from build123d import *

# Parameters (mm, degrees)
SKETCH1_R               = 10
SKETCH1_R_2             = 6
BOSS_EXTRUDE1_DEPTH     = 3
SKETCH2_R               = 1.5
CUT_EXTRUDE1_DEPTH      = 4
CUT_EXTRUDE1_DEPTH_BACK = 4
F_4_0MM_DOWEL_HOLE1_D   = 4


with BuildPart() as part:
    # Sketch1 → Boss-Extrude1 (new body, symmetric)
    with BuildSketch(Plane(origin=(0, 0, 0), x_dir=(0, 0, -1), z_dir=(1, 0, 0))):
        Circle(SKETCH1_R)
        with BuildLine():
            ThreePointArc((40.6, -5.969924623), (34, 0), (40.6, 5.969924623))
            Line((40.6, 5.969924623), (1, 9.949874371))
            ThreePointArc((1, 9.949874371), (7.416198487, 6.708203932), (10, 0))
            ThreePointArc((10, 0), (7.416198487, -6.708203933), (1, -9.949874371))
            Line((1, -9.949874371), (40.6, -5.969924623))
        make_face()
        with Locations((40, 0)):
            Circle(SKETCH1_R_2)
    extrude(amount=BOSS_EXTRUDE1_DEPTH, both=True)

    # Sketch2 → Cut-Extrude1 (cut, two sides)
    with BuildSketch(Plane(origin=(0, 0, 0), x_dir=(0, 0, -1), z_dir=(1, 0, 0))) as cut_extrude1_sk:
        with Locations((4.949747468, 4.949747468)):
            Circle(SKETCH2_R)
        with Locations((4.949747468, -4.949747468)):
            Circle(SKETCH2_R)
        with Locations((-4.949747468, -4.949747468)):
            Circle(SKETCH2_R)
        with Locations((-4.949747468, 4.949747468)):
            Circle(SKETCH2_R)
    extrude(amount=CUT_EXTRUDE1_DEPTH, mode=Mode.SUBTRACT)
    extrude(cut_extrude1_sk.sketch, amount=-CUT_EXTRUDE1_DEPTH_BACK, mode=Mode.SUBTRACT)

    # 4.0mm Dowel Hole1 (through all)
    with Locations(Plane(origin=(3, 0, 0), x_dir=(0, 0, -1), z_dir=(1, 0, 0))):
        with Locations((40, 0)):
            Hole(F_4_0MM_DOWEL_HOLE1_D / 2)


solid = part.part
Input: part model. Units: mm. Frame: model coordinates. Round coordinates to 2 decimals unless told otherwise and drop trailing zeros. Order: outer loops, then holes, each group sorted by start corner. A loop starts at its lowest first (then second) coordinate and runs counter-clockwise, first axis right, second up.
1. Cut plane A-A, the plane y = 0. Output: boundary loops of the cut face in (x, z), then the cut area to 3 significant figures.
The answers:
outline: (-3, -46) - (3, -46) - (3, -42) - (-3, -42) - close; (-3, -38) - (3, -38) - (3, 10) - (-3, 10) - close
area: 312 mm2
2. Cut plane D-D, the plane x = 2.5. Output: boundary loops of the cut face in (y, z), then the cut area to 3 significant figures.
The answers:
outline: (-9.95, -1) - (-5.97, -40.6) arc R6 ccw to (5.97, -40.6) - (9.95, -1) arc R10 ccw (long way) to start; hole circle Ø3 at (-4.95, -4.95); hole circle Ø3 at (-4.95, 4.95); hole circle Ø4 at (0, -40); hole circle Ø3 at (4.95, -4.95); hole circle Ø3 at (4.95, 4.95)
area: 816 mm2
3. Cut plane B-B, the plane y = -4. Output: boundary loops of the cut face in (x, z), then the cut area to 3 significant figures.
The answers:
outline: (-3, -44.47) - (3, -44.47) - (3, -6.11) - (-3, -6.11) - close; (-3, -3.79) - (3, -3.79) - (3, 3.79) - (-3, 3.79) - close; (-3, 6.11) - (3, 6.11) - (3, 9.17) - (-3, 9.17) - close
area: 294 mm2
4. Material intervals for line 1 (Z direction, x = -2, y = 4.75); line 2 (Z direction, x = -1.75, y = 4); line 3 (Y direction, x = 2.75, z = -41.5), sorted ascending.
The answers:
line 1: z = -43.67 to -6.44, -3.46 to 3.46, 6.44 to 8.8
line 2: z = -44.47 to -6.11, -3.79 to 3.79, 6.11 to 9.17
line 3: y = -5.81 to -1.32, 1.32 to 5.81
5. Pin query (flat end, axial travel): P1, Ø3, axis at x = 2, z = -7, coming from the +Y side; P2, Ø3, axis at x = 1.5, y = 4, coming from the -Z side; P3, Ø1.5, axis at x = -2, y = 1.5, coming from the +Z side. Return the tip coordinate at first contact, or that it passes through.
The answers:
P1: stops at y = 9.5
P2: stops at z = -45.45
P3: stops at z = 9.97
6. Cut plane C-C, the plane z = -40. Output: boundary loops of the cut face in (x, y), then the cut area to 3 significant figures.
The answers:
outline: (-3, -6.03) - (3, -6.03) - (3, -2) - (-3, -2) - close; (-3, 2) - (3, 2) - (3, 6.03) - (-3, 6.03) - close
area: 48.4 mm2
7. Mould query, pull axis Z, two halves, no side actions, for faces 1 (the face through (-3, 0, -18)), 2 (the face through (0, 0, -46)), 3 (the face through (0.042, -3.685, -5.756)). Classes: released by +Z, released by -Z, zero draft, split by the parting line, or undercut.
The answers:
face 1: zero draft
face 2: released by -Z
face 3: undercut
